from build123d import *

# Parameters (mm, degrees)
F1_DEPTH = 8
F3_D     = 6.6


with BuildPart() as f1:
    # F0 (on Front) → F1 (new body)
    with BuildSketch(Plane.XZ):
        with BuildLine():
            Line((40, 22.5), (-40, 22.5))
            Line((-40, 22.5), (-40, -22.5))
            Line((-40, -22.5), (-10.1, -22.5))
            Line((-10.1, -22.5), (-10.1, -2.5))
            ThreePointArc((-10.1, -2.5), (0, 7.6), (10.1, -2.5))
            Line((10.1, -2.5), (10.1, -22.5))
            Line((10.1, -22.5), (40, -22.5))
            Line((40, -22.5), (40, 22.5))
        make_face()
    extrude(amount=F1_DEPTH)

    # F3 (through all)
    with Locations(Plane.XZ.offset(8)):
        with Locations((-34, 16.5), (-34, -16.5), (34, -16.5), (34, 16.5)):
            Hole(F3_D / 2)


solid = f1.part
Geometry: final body of the model. Coordinates: model frame, mm. A direction names the side the tool comes from. Round coordinates to 2 decimals unless told otherwise and drop trailing zeros. Loops run counter-clockwise (first coordinate to the right, second up) from the corner with the lowest first, then second, coordinate; pieces in that order, holes last. Notation, with made-up numbers: (21, 13) -> (52, 13) arc R31 cw to (52, 43) -> close; hole circle Ø9 at (2, -12.75). An arc over 180 degrees is marked (long way). One line per question, with ' | ' between items. Start each with the question number.
1. Section A-A on z = 16.5. Output: boundary loops of the cut face in (x, y).
2. Section D-D on z = -16.5. Output: boundary loops of the cut face in (x, y), and give its area (3 significant figures).
3. Contact query for flat-ended pins moving along their axis: pin 1 (5.5 mm diameter, centred on x = 34, z = 16.5, fed in from -Y); pin 2 (10 mm diameter, centred on x = 25, z = 15, fed in from +Y). Output: stop coordinate, or through.
4. Line query: line 1 along Z through (x, y) = (34, -3.75); line 2 along X through (y, z) = (-0.25, -10.5); line 3 along X through (y, z) = (-6.75, -19). Output: solid intervals per line, ascending. Write a range as [from, to].
5. Mould query, pull axis X, two halves, no side actions, for faces 3 (the face through (-40, -4, 0)), 4 (the face through (-0.2, -3.9, 7.6)), 5 (the face through (1, -4, 22.5)). Classes: pulls with the +X half, pulls with the -X half, needs draft (parallel to the pull), parting line crosses it, or undercut.
6. Set-up query: faces 1 (the face through (-10.1, -4, -13)), 2 (the face through (-25, -4, -22.5)). Return all of +Z, -Z, +X, -X, +Y, -Y with unobstructed straight access to the full face (end or side cutting, diameter ignored); none if empty.
7. Section C-C on y = -1.75. Output: boundary loops of the cut face in (x, z).
8. Section B-B on x = -34. Output: boundary loops of the cut face in (y, z).
Returned:
1) outline: (-40, -8) -> (-37.3, -8) -> (-37.3, 0) -> (-40, 0) -> close; (-30.7, -8) -> (30.7, -8) -> (30.7, 0) -> (-30.7, 0) -> close; (37.3, -8) -> (40, -8) -> (40, 0) -> (37.3, 0) -> close
2) outline: (-40, -8) -> (-37.3, -8) -> (-37.3, 0) -> (-40, 0) -> close; (-30.7, -8) -> (-10.1, -8) -> (-10.1, 0) -> (-30.7, 0) -> close; (10.1, -8) -> (30.7, -8) -> (30.7, 0) -> (10.1, 0) -> close; (37.3, -8) -> (40, -8) -> (40, 0) -> (37.3, 0) -> close | area: 373 mm2
3) pin 1: passes through | pin 2: stops at y = 0
4) line 1: z = [-22.5, -19.8], [-13.2, 13.2], [19.8, 22.5] | line 2: x = [-40, -10.1], [10.1, 40] | line 3: x = [-40, -36.15], [-31.85, -10.1], [10.1, 31.85], [36.15, 40]
5) face 3: pulls with the -X half | face 4: undercut | face 5: needs draft
6) face 1: -Z, +Y, -Y | face 2: -Z, +X, -X, +Y, -Y
7) outline: (-40, -22.5) -> (-10.1, -22.5) -> (-10.1, -2.5) arc R10.1 cw to (10.1, -2.5) -> (10.1, -22.5) -> (40, -22.5) -> (40, 22.5) -> (-40, 22.5) -> close; hole circle Ø6.6 at (-34, -16.5); hole circle Ø6.6 at (-34, 16.5); hole circle Ø6.6 at (34, -16.5); hole circle Ø6.6 at (34, 16.5)
8) outline: (-8, -22.5) -> (0, -22.5) -> (0, -19.8) -> (-8, -19.8) -> close; (-8, -13.2) -> (0, -13.2) -> (0, 13.2) -> (-8, 13.2) -> close; (-8, 19.8) -> (0, 19.8) -> (0, 22.5) -> (-8, 22.5) -> close
